For this review, take the finished solid that the model builds, in its own axes (mm). Coordinates: 2 decimals unless noted, no trailing zeros. Write each loop counter-clockwise with the first axis right and the second up, starting at its lowest first coordinate (ties: lowest second). Pieces come first, ordered by that corner, then holes. Notation, with made-up numbers: (-29.75, 50.5) -> (-23.75, 50.5) arc R9 cw to (-23.75, 54.5) -> close; hole circle Ø6 at (-8.75, 39). An arc over 180 degrees is marked (long way). One line per item, written item: value. Start each with the question number.
1) For pin 1 Ø0.9 at (x, y) = (-16, -8) entering from -Z; pin 2 Ø0.8 at (y, z) = (-34, 1) entering from -X; pin 3 Ø0.8 at (y, z) = (-34, 1) entering from +X; pin 4 Ø0.8 at (x, y) = (-11.43, 28.12) entering from -Z, all flat-tipped, find the tip position at first contact; note any pin that passes through.
2) Add section A-A (x = -11.43). State the section outline as (y, z) points.
3) Add section B-B (z = 1.1). State the section outline as (x, y) points (3 decimals), and give its area (3 significant figures).
4) For probe 1 along Y at (x, z) = (-11.43, 1); probe 2 along X at (y, z) = (-27, 1.3) (3 decimals); probe 3 along Y at (x, z) = (-16, 1), list the stretches that pass through material, from the lowest coordinate up. Write a range as from..to.
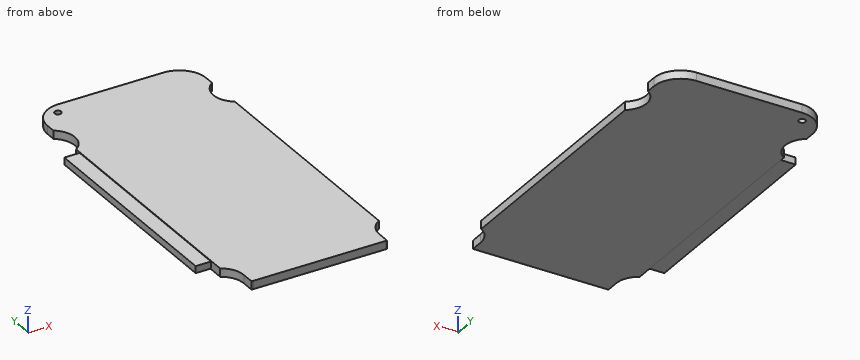
from build123d import *

# Parameters (mm, degrees)
F0_W      = 30.19
F0_H      = 57
F1_DEPTH  = 1.5748
F2_W      = 30.19
F2_H      = 1.5748
F3_DEPTH  = 6.8834
F4_R      = 2.54
F5_R      = 4.32816
F6_DEPTH  = 1.5758
F7_W      = 30.19
F7_H      = 1.5748
F8_DEPTH  = 1.905
F9_R      = 5.08
F10_R     = 0.635
F11_DEPTH = 25.4
F12_W     = 41.4245947965
F12_H     = 1.3208
F13_DEPTH = 2.921


with BuildPart() as f1:
    # F0 (on Top) → F1 (new body)
    with BuildSketch(Plane.XY):
        Rectangle(F0_W, F0_H)
    extrude(amount=F1_DEPTH)

    # F2 (on face) → F3 (join)
    with BuildSketch(Plane.XZ.offset(28.5)):
        with Locations((0, 0.7874)):
            Rectangle(F2_W, F2_H)
    extrude(amount=F3_DEPTH)

    # F4
    f4_edges = [f1.edges().sort_by_distance(p)[0] for p in [
        (15.095, -35.3834, 0.7874),
        (-15.095, -35.3834, 0.7874),
    ]]
    fillet(f4_edges, radius=F4_R)

    # F5 (on face) → F6 (cut, through all)
    with BuildSketch(Plane.XY.offset(1.5748)):
        with Locations((-17.51457, 19.8616)):
            Circle(F5_R)
        with Locations((17.51457, 19.8616)):
            Circle(F5_R)
        with BuildLine():
            Line((-17.2212, -32.9196), (-12.89304, -32.9196))
            ThreePointArc((-12.89304, -32.9196), (-20.2816712861, -29.8591287139), (-17.2212, -37.24776))
            Line((-17.2212, -37.24776), (-17.2212, -32.9196))
        make_face()
        with BuildLine():
            Line((-12.89304, -37.24776), (-12.89304, -32.9196))
            ThreePointArc((-12.89304, -32.9196), (-14.1607287139, -35.9800712861), (-17.2212, -37.24776))
            Line((-17.2212, -37.24776), (-12.89304, -37.24776))
        make_face()
        with BuildLine():
            ThreePointArc((-17.2212, -37.24776), (-14.1607287139, -35.9800712861), (-12.89304, -32.9196))
            Line((-12.89304, -32.9196), (-17.2212, -32.9196))
            Line((-17.2212, -32.9196), (-17.2212, -37.24776))
        make_face()
        with BuildLine():
            ThreePointArc((17.2212, -37.24776), (20.2816712861, -35.9800712861), (21.54936, -32.9196))
            ThreePointArc((21.54936, -32.9196), (17.2212, -28.59144), (12.89304, -32.9196))
            Line((12.89304, -32.9196), (17.2212, -32.9196))
            Line((17.2212, -32.9196), (17.2212, -37.24776))
        make_face()
        with BuildLine():
            Line((17.2212, -32.9196), (12.89304, -32.9196))
            ThreePointArc((12.89304, -32.9196), (14.1607287139, -35.9800712861), (17.2212, -37.24776))
            Line((17.2212, -37.24776), (17.2212, -32.9196))
        make_face()
        with BuildLine():
            ThreePointArc((17.2212, -37.24776), (14.1607287139, -35.9800712861), (12.89304, -32.9196))
            Line((12.89304, -32.9196), (12.89304, -37.24776))
            Line((12.89304, -37.24776), (17.2212, -37.24776))
        make_face()
    extrude(amount=-F6_DEPTH, mode=Mode.SUBTRACT)

    # F7 (on face) → F8 (join)
    with BuildSketch(Plane(origin=(0, 28.5, 0), x_dir=(-1, 0, 0), z_dir=(0, 1, 0))):
        with Locations((0, 0.7874)):
            Rectangle(F7_W, F7_H)
    extrude(amount=F8_DEPTH)

    # F9
    f9_edges = [f1.edges().sort_by_distance(p)[0] for p in [
        (-15.095, 30.405, 0.7874),
        (15.095, 30.405, 0.7874),
    ]]
    fillet(f9_edges, radius=F9_R)

    # F10 (on face) → F11 (cut)
    with BuildSketch(Plane.XY.offset(1.5748)):
        with Locations((-11.43, 28.1166)):
            Circle(F10_R)
    extrude(amount=-F11_DEPTH, mode=Mode.SUBTRACT)

    # F12 (on face) → F13 (join)
    with BuildSketch(Plane(origin=(-15.095, 0, 0), x_dir=(0, -1, 0), z_dir=(-1, 0, 0))):
        with Locations((5.5271026017, 0.7874)):
            Rectangle(F12_W, F12_H)
    extrude(amount=F13_DEPTH)


solid = f1.part
Numbers:
1. pin 1: z = 0.13
1. pin 2: x = -12.89
1. pin 3: x = 12.89
1. pin 4: through
2. outline: (-35.38, 0) -> (27.48, 0) -> (27.48, 1.57) -> (-35.38, 1.57) -> close; (28.75, 0) -> (30.2, 0) -> (30.2, 1.57) -> (28.75, 1.57) -> close
3. outline: (-18.016, -26.239) -> (-15.095, -26.239) -> (-15.095, -29.15) arc R4.328 cw to (-12.893, -32.92) -> (-12.893, -35.361) arc R2.54 ccw to (-12.555, -35.383) -> (12.555, -35.383) arc R2.54 ccw to (12.893, -35.361) -> (12.893, -32.92) arc R4.328 cw to (15.095, -29.15) -> (15.095, 16.273) arc R4.328 cw to (15.095, 23.45) -> (15.095, 25.325) arc R5.08 ccw to (10.015, 30.405) -> (-10.015, 30.405) arc R5.08 ccw to (-15.095, 25.325) -> (-15.095, 23.45) arc R4.328 cw to (-15.095, 16.273) -> (-15.095, 15.185) -> (-18.016, 15.185) -> close; hole circle Ø1.27 at (-11.43, 28.117)
3. area: 2,050 mm²
4. probe 1: -35.38..27.48, 28.75..30.2
4. probe 2: -15.095..15.095
4. probe 3: -26.24..15.19
